```python
from build123d import *

# Parameters (mm, degrees)
F0_W     = 393.7
F0_H     = 393.7
F0_W_2   = 317.5
F0_H_2   = 317.5
F1_DEPTH = 38.1
F2_W     = 38.1
F2_H     = 38.1
F3_DEPTH = 508
F4_W     = 317.5
F4_H     = 317.5
F5_DEPTH = 38.1


with BuildPart() as f1:
    # F0 (on Top) → F1 (new body)
    with BuildSketch(Plane.XY):
        Rectangle(F0_W, F0_H)
        Rectangle(F0_W_2, F0_H_2, mode=Mode.SUBTRACT)
    extrude(amount=F1_DEPTH)

    # F2 (on face) → F3 (join)
    with BuildSketch(Plane(origin=(0, 0, 0), x_dir=(1, 0, 0), z_dir=(0, 0, -1))):
        with Locations((-177.8, 177.8)):
            Rectangle(F2_W, F2_H)
        with Locations((-177.8, -177.8)):
            Rectangle(F2_W, F2_H)
        with Locations((177.8, 177.8)):
            Rectangle(F2_W, F2_H)
        with Locations((177.8, -177.8)):
            Rectangle(F2_W, F2_H)
    extrude(amount=F3_DEPTH)

    # F4 (on face) → F5 (join)
    with BuildSketch(Plane(origin=(0, 0, -508), x_dir=(1, 0, 0), z_dir=(0, 0, -1))):
        Polygon((158.75, -196.85), (196.85, -196.85), (196.85, -158.75), (196.85, 158.75), (196.85, 196.85), (158.75, 196.85), (-158.75, 196.85), (-196.85, 196.85), (-196.85, 158.75), (-196.85, -158.75), (-196.85, -196.85), (-158.75, -196.85), align=None)
        Rectangle(F4_W, F4_H, mode=Mode.SUBTRACT)
    extrude(amount=F5_DEPTH)


solid = f1.part
```
Source: CAD feature listing. Evaluate the final solid. Frame: model axes, mm. A direction names the side the tool comes from. Round coordinates to 2 decimals unless told otherwise and drop trailing zeros. Loops run counter-clockwise (first coordinate to the right, second up) from the corner with the lowest first, then second, coordinate; pieces in that order, holes last.
(1) Section query A-A (x = -150.5). Output: boundary loops of the cut face in (y, z).
From the geometry:
outline: (-196.85, -546.1) - (-158.75, -546.1) - (-158.75, -508) - (-196.85, -508) - close; (-196.85, 0) - (-158.75, 0) - (-158.75, 38.1) - (-196.85, 38.1) - close; (158.75, -546.1) - (196.85, -546.1) - (196.85, -508) - (158.75, -508) - close; (158.75, 0) - (196.85, 0) - (196.85, 38.1) - (158.75, 38.1) - close
(2) Material intervals for probe 1 along Z at (x, y) = (-60.5, 161); probe 2 along X at (y, z) = (-165, -162.5), sorted ascending.
From the geometry:
probe 1: z = -546.1 to -508, 0 to 38.1
probe 2: x = -196.85 to -158.75, 158.75 to 196.85
(3) Section query C-C (x = 166). Output: boundary loops of the cut face in (y, z), and give its area (3 significant figures).
From the geometry:
outline: (-196.85, -546.1) - (196.85, -546.1) - (196.85, 38.1) - (-196.85, 38.1) - close; hole (-158.75, -508) - (158.75, -508) - (158.75, 0) - (-158.75, 0) - close
area: 68,700 mm2
(4) Pull-direction query (Y, two-part tool) for faces 6 (the flat face through (158.75, 178, -250)), 7 (the flat face through (178, 2, 0)); classes: +Y half, -Y half, draft (parallel to the pull), parting line (faces both ways), or undercut.
From the geometry:
face 6: draft
face 7: undercut
(5) Access query for faces 1 (the flat face through (-2, -178, 0)), 2 (the flat face through (-178, -158.75, -250)), 3 (the flat face through (-178, 3, 38.1)), 4 (the flat face through (196.85, 178, -250)), 5 (the flat face through (-2, 158.75, 19)). Directions: +Z, -Z, +X, -X, +Y, -Y. A direction counts if a zero-diameter tool reaches every point of the face in a straight line with its end or side. Return the directions, or none.
From the geometry:
face 1: +Y, -Y
face 2: +X, -X
face 3: +Z, +X, -X, +Y, -Y
face 4: +Z, -Z, +X, +Y, -Y
face 5: +Z, -Z
